from build123d import *

# Parameters (mm, degrees)
SKETCH1_R               = 3
SKETCH1_R_2             = 16.15
BOSS_EXTRUDE1_DEPTH     = 10
CUT_EXTRUDE1_DEPTH      = 36
CUT_EXTRUDE1_DEPTH_BACK = 36
CUT_EXTRUDE2_DEPTH      = 4.263908078
CUT_EXTRUDE2_DEPTH_BACK = 7.736091922
CUT_EXTRUDE3_DEPTH      = 4.263908078
CUT_EXTRUDE3_DEPTH_BACK = 7.736091922
FILLET1_R               = 1.5


with BuildPart() as part:
    # Sketch1 → Boss-Extrude1 (new body)
    with BuildSketch(Plane.XY):
        Polygon((-72, 16.21061599), (-72, -16.21061599), (-53.874481608, -25.873120341), (-18.780890439, -27.25079114), (-7.646290238, -32.818629475), (0, -35), (6.138156767, -35), (72, -16.21061599), (72, 16.21061599), (6.138156767, 35), (0, 35), (-7.646290238, 32.818629475), (-18.780890439, 27.25079114), (-53.874481608, 25.873120341), align=None)
        with Locations((0, 30)):
            Circle(SKETCH1_R, mode=Mode.SUBTRACT)
        with Locations((-50, 0)):
            Circle(SKETCH1_R_2, mode=Mode.SUBTRACT)
        with Locations((0, -30)):
            Circle(SKETCH1_R, mode=Mode.SUBTRACT)
        with Locations((50, 0)):
            Circle(SKETCH1_R_2, mode=Mode.SUBTRACT)
    extrude(amount=BOSS_EXTRUDE1_DEPTH)

    # Sketch2 → Cut-Extrude1 (cut, two sides)
    with BuildSketch(Plane(origin=(0, 0, 0), x_dir=(1, 0, 0), z_dir=(0, 1, 0))) as cut_extrude1_sk:
        Polygon((-30, -10), (-24.053688771, -6.736091922), (4.484766303, -6.736091922), (24.053688771, -6.736091922), (30, -10), align=None)
        Polygon((-72, 0), (-72, -4.2256576), (-37.698462898, -4.2256576), (-30, 0), align=None)
        Polygon((30, 0), (72, 0), (72, -4.2256576), (37.698462898, -4.2256576), align=None)
    extrude(amount=CUT_EXTRUDE1_DEPTH, mode=Mode.SUBTRACT)
    extrude(cut_extrude1_sk.sketch, amount=-CUT_EXTRUDE1_DEPTH_BACK, mode=Mode.SUBTRACT)

    # Sketch3 → Cut-Extrude2 (cut, two sides)
    with BuildSketch(Plane.XY.offset(6.736091922)) as cut_extrude2_sk:
        Polygon((5.2, -10.7), (-5.2, -10.7), (-5.2, 7.758003241), (-2.908652734, 10.7), (2.908652734, 10.7), (5.2, 7.758003241), align=None)
    extrude(amount=CUT_EXTRUDE2_DEPTH, mode=Mode.SUBTRACT)
    extrude(cut_extrude2_sk.sketch, amount=-CUT_EXTRUDE2_DEPTH_BACK, mode=Mode.SUBTRACT)

    # Sketch4 → Cut-Extrude3 (cut, two sides)
    with BuildSketch(Plane.XY.offset(6.736091922)) as cut_extrude3_sk:
        Polygon((-18.641801382, 13.783435693), (-18.641801382, -13.783435693), (-12.900018937, -22.526604416), (-12.900018937, 22.526604416), align=None)
        Polygon((18.641801382, 13.783435693), (12.900018937, 22.526604416), (12.900018937, -22.526604416), (18.641801382, -13.783435693), align=None)
    extrude(amount=CUT_EXTRUDE3_DEPTH, mode=Mode.SUBTRACT)
    extrude(cut_extrude3_sk.sketch, amount=-CUT_EXTRUDE3_DEPTH_BACK, mode=Mode.SUBTRACT)

    # Fillet1
    fillet1_edges = [part.edges().sort_by_distance(p)[0] for p in [
        (-12.900018937, -22.526604416, 3.368045961),
        (-18.641801382, -13.783435693, 3.368045961),
        (-18.641801382, 13.783435693, 3.368045961),
        (-12.900018937, 22.526604416, 3.368045961),
        (18.641801382, 13.783435693, 3.368045961),
        (12.900018937, -22.526604416, 3.368045961),
        (12.900018937, 22.526604416, 3.368045961),
    ]]
    fillet(fillet1_edges, radius=FILLET1_R)


solid = part.part
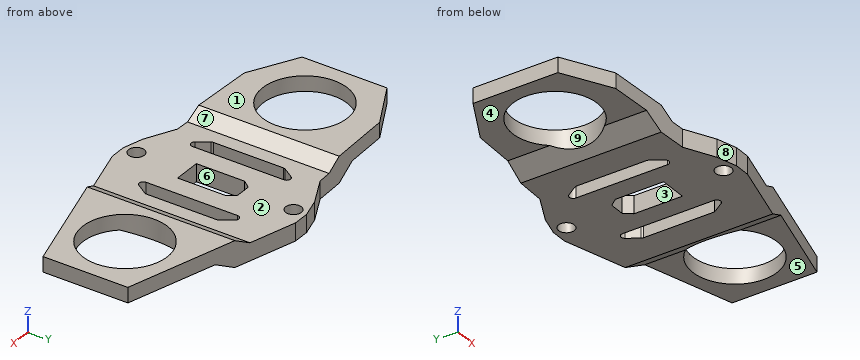
Input: part model. Units: mm. Frame: model coordinates. Face numbers are marked on the shaded views. A direction names the side the tool comes from. Coordinates: 2 decimals unless noted, no trailing zeros. Loops run counter-clockwise (first coordinate to the right, second up) from the corner with the lowest first, then second, coordinate; pieces in that order, holes last.
(1) Set-up query: the marked faces 1, 2, 3, 4 and 5. Return all of +Z, -Z, +X, -X, +Y, -Y with unobstructed straight access to the full face (end or side cutting, diameter ignored); none if empty.
(2) First-contact query: pin 1 Ø2 at (y, z) = (2, 3) entering from +X; pin 2 Ø5 at (x, z) = (-42.5, 2) entering from +Y; pin 3 Ø24 at (x, y) = (3, 3) entering from +Z. Flat tips, straight axial feed; report the tip coordinate or a pass-through.
(3) Section B-B on x = 50. Return the cut outline in (y, z), then the cut area to 3 significant figures.
(4) Section A-A on y = 0. Count the separate pieces of the cut face and the enclosed holes in it, then the cut area to 3 significant figures.
(5) Material intervals for probe 1 along Y at (x, z) = (0, 4.75); probe 2 along X at (y, z) = (4, 4); probe 3 along X at (y, z) = (0, 8), sorted ascending.
(6) Section C-C on x = -36. Return the cut outline in (y, z), then the cut area to 3 significant figures.
(7) Pull-direction query (Y, two-part tool) for the marked faces 6, 7, 8 and 9; classes: released by +Y, released by -Y, zero draft, split by the parting line, or undercut.
Data:
1. face 1: +Z, +X, -X, +Y, -Y
1. face 2: +Z, +Y, -Y
1. face 3: +Z, -Z
1. face 4: -Z, -X, +Y, -Y
1. face 5: -Z, +X, +Y, -Y
2. pin 1: stops at x = 34.13
2. pin 2: stops at y = 26.36
2. pin 3: stops at z = 6.74
3. outline: (-22.49, 4.23) - (-16.15, 4.23) - (-16.15, 10) - (-22.49, 10) - close; (16.15, 4.23) - (22.49, 4.23) - (22.49, 10) - (16.15, 10) - close
3. area: 73.2 mm2
4. separate pieces: 6
4. enclosed holes: 0
4. area: 413 mm2
5. probe 1: y = -35 to -33, -27 to -10.7, 10.7 to 27, 33 to 35
5. probe 2: x = -34.35 to -18.64, -12.9 to -5.2, 5.2 to 12.9, 18.64 to 34.35
5. probe 3: x = -72 to -66.15, -33.85 to -26.36, 26.36 to 33.85, 66.15 to 72
6. outline: (-26.57, 3.29) - (-8.05, 3.29) - (-8.05, 10) - (-26.57, 10) - close; (8.05, 3.29) - (26.57, 3.29) - (26.57, 10) - (8.05, 10) - close
6. area: 248 mm2
7. face 6: undercut
7. face 7: zero draft
7. face 8: released by -Y
7. face 9: undercut
